from build123d import *

# Parameters (mm, degrees)
F0_W     = 20
F0_H     = 12
F1_DEPTH = 40
F3_DEPTH = 16
F5_D     = 5


with BuildPart() as f1:
    # F0 (on Front) → F1 (new body)
    with BuildSketch(Plane.XZ):
        Rectangle(F0_W, F0_H)
    extrude(amount=F1_DEPTH)

    # F2 (on face) → F3 (cut)
    with BuildSketch(Plane.XY.offset(6)):
        with BuildLine():
            Line((10, 0), (-10, 0))
            ThreePointArc((-10, 0), (0, -2.182576), (10, 0))
        make_face()
        with BuildLine():
            Line((-10, -40), (10, -40))
            ThreePointArc((10, -40), (0, -37.655644), (-10, -40))
        make_face()
    extrude(amount=-F3_DEPTH, mode=Mode.SUBTRACT)

    # F5 (through all)
    with Locations(Plane(origin=(0, 0, 0), x_dir=(1, 0, 0), z_dir=(0, 1, 0))):
        with Locations((0, 0)):
            Hole(F5_D / 2)


solid = f1.part
For this review, take the finished solid that the model builds, in its own axes (mm). Round coordinates to 2 decimals unless told otherwise and drop trailing zeros. Order: outer loops, then holes, each group sorted by start corner. A loop starts at its lowest first (then second) coordinate and runs counter-clockwise, first axis right, second up. Notation, with made-up numbers: (44, -25.5) -> (64, -25.5) arc R19 ccw to (64, -10.5) -> close; hole circle Ø11 at (59, 14). An arc over 180 degrees is marked (long way). Put each result on its own line as item: value.
Q1. Add section C-C on y = -34.5. Write out the cut boundary in (x, z), plus the area to 3 significant figures.
Check result:
outline: (-10, -6) -> (10, -6) -> (10, 6) -> (-10, 6) -> close; hole circle Ø5 at (0, 0)
area: 220 mm2
Q2. Add section B-B on x = 0. Write out the cut boundary in (y, z).
Check result:
outline: (-37.66, -6) -> (-2.18, -6) -> (-2.18, -2.5) -> (-37.66, -2.5) -> close; (-37.66, 2.5) -> (-2.18, 2.5) -> (-2.18, 6) -> (-37.66, 6) -> close
Q3. Insertion check: pin 1 Ø1.5 at (x, z) = (4, 0) entering from +Y; pin 2 Ø4 at (x, z) = (0, 0) entering from -Y; pin 3 Ø2 at (x, z) = (-5, -4) entering from +Y. Each pin has a flat end and moves straight along its axis. Give the tip position at first contact, or say it passes through.
Check result:
pin 1: y = -1.71
pin 2: through
pin 3: y = -1.42
Q4. For probe 1 along Z at (x, y) = (0, -9.5); probe 2 along X at (y, z) = (-14, -1); probe 3 along Z at (x, y) = (-1, -23.5), list the stretches that pass through material, from the lowest coordinate up. Write a range as [from, to].
Check result:
probe 1: [-6, -2.5], [2.5, 6]
probe 2: [-10, -2.29], [2.29, 10]
probe 3: [-6, -2.29], [2.29, 6]
Q5. Add section A-A on z = 0. Write out the cut boundary in (x, y).
Check result:
outline: (-10, -40) arc R22.5 cw to (-2.5, -37.79) -> (-2.5, -2.05) arc R24 cw to (-10, 0) -> close; (2.5, -37.79) arc R22.5 cw to (10, -40) -> (10, 0) arc R24 cw to (2.5, -2.05) -> close
Q6. Add section D-D on z = 3.5. Write out the cut boundary in (x, y), plus the area to 3 significant figures.
Check result:
outline: (-10, -40) arc R22.5 cw to (10, -40) -> (10, 0) arc R24 cw to (-10, 0) -> close
area: 739 mm2
Q7. Mouldability with a two-part tool opening along X and no side actions: class faces 1 (the flat face through (-10, -20, 0)), 2 (the cylindrical face through (0.54, -20.17, 2.44)), 3 (the flat face through (10, -20, 0)), 4 (the flat face through (0, -20, -6)) as pulls with the +X half, pulls with the -X half, needs draft (parallel to the pull), parting line crosses it, or undercut.
Check result:
face 1: pulls with the -X half
face 2: undercut
face 3: pulls with the +X half
face 4: needs draft
